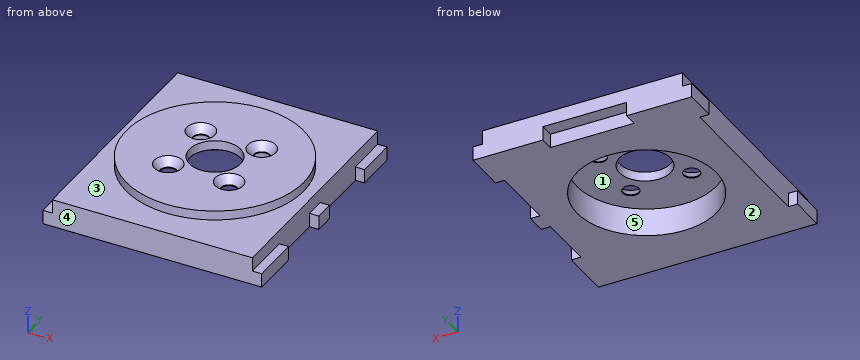
from build123d import *

# Parameters (mm, degrees)
F0_R     = 15
F1_DEPTH = 3
F2_R     = 15
F2_W     = 18
F2_H     = 3
F3_DEPTH = 3
F4_R     = 19.092503
F4_R_2   = 1.75
F4_R_3   = 5.5
F5_DEPTH = 2
F6_SIZE2 = 1.8
F6_SIZE  = 1.25
F7_W     = 2
F7_H     = 0.1
F8_DEPTH = 3.001


with BuildPart() as f1:
    # F0 (on Top) → F1 (new body)
    with BuildSketch(Plane.XY):
        Polygon((-9.5, 25.15), (-23.5, 25.15), (-23.5, 18.15), (-21.5, 18.15), (-21.5, -17.35), (-23.5, -17.35), (-23.5, -25.15), (23.5, -25.15), (23.5, -14.35), (21.5, -14.35), (21.5, -2.35), (23.5, -2.35), (23.5, 2.15), (21.5, 2.15), (21.5, 16.15), (23.5, 16.15), (23.5, 25.15), (8.5, 25.15), (8.5, 22.15), (-9.5, 22.15), align=None)
        with Locations((-0.135, -0.392646)):
            Circle(F0_R, mode=Mode.SUBTRACT)
    extrude(amount=F1_DEPTH)

    # F2 (on face) → F3 (join)
    with BuildSketch(Plane.XY.offset(3)):
        Polygon((-21.5, 25.15), (-21.5, 18.15), (-21.5, -17.35), (-21.5, -25.15), (21.5, -25.15), (21.5, -14.35), (21.5, -2.35), (21.5, 2.15), (21.5, 16.15), (21.5, 25.15), (8.5, 25.15), (8.5, 22.15), (-9.5, 22.15), (-9.5, 25.15), align=None)
        with Locations((-0.135, -0.392646)):
            Circle(F2_R, mode=Mode.SUBTRACT)
        with Locations((-0.5, 23.65)):
            Rectangle(F2_W, F2_H)
    extrude(amount=F3_DEPTH)

    # F4 (on face) → F5 (join)
    with BuildSketch(Plane.XY.offset(6)):
        Circle(F4_R)
        with Locations((-6.540738, -6.540738)):
            Circle(F4_R_2, mode=Mode.SUBTRACT)
        with Locations((6.540738, -6.540738)):
            Circle(F4_R_2, mode=Mode.SUBTRACT)
        with Locations((-6.540738, 6.540738)):
            Circle(F4_R_2, mode=Mode.SUBTRACT)
        Circle(F4_R_3, mode=Mode.SUBTRACT)
        with Locations((6.540738, 6.540738)):
            Circle(F4_R_2, mode=Mode.SUBTRACT)
    extrude(amount=F5_DEPTH)

    # F6
    f6_edges = [f1.edges().sort_by_distance(p)[0] for p in [
        (-8.290738, 6.540738, 8),
        (4.790738, 6.540738, 8),
        (4.790738, -6.540738, 8),
        (-8.290738, -6.540738, 8),
    ]]
    chamfer(f6_edges, length=F6_SIZE, length2=F6_SIZE2)

    # F7 (on face) → F8 (cut, through all)
    with BuildSketch(Plane.XY.offset(3)):
        with Locations((22.5, 2.1)):
            Rectangle(F7_W, F7_H)
        with Locations((22.5, -2.3)):
            Rectangle(F7_W, F7_H)
    extrude(amount=-F8_DEPTH, mode=Mode.SUBTRACT)


solid = f1.part
Read the model definition and answer for the solid it produces. Units are mm, in the model's axes. Face numbers are marked on the shaded views. A direction names the side the tool comes from. Coordinates: 2 decimals unless noted, no trailing zeros. Loops run counter-clockwise (first coordinate to the right, second up) from the corner with the lowest first, then second, coordinate; pieces in that order, holes last. Notation, with made-up numbers: (28.5, -12) - (49.5, -12) arc R30 cw to (49.5, 21) - close; hole circle Ø9 at (64.25, -25.5). An arc over 180 degrees is marked (long way). Answer in a Markdown table with one row per item.
Q1. Find section D-D on x = 0. Write down the section's boundary in (y, z).
Here are the results:
| item | result |
|---|---|
| outline | (-25.15, 0) - (-15.39, 0) - (-15.39, 6) - (-5.5, 6) - (-5.5, 8) - (-19.09, 8) - (-19.09, 6) - (-25.15, 6) - close; (5.5, 6) - (14.61, 6) - (14.61, 0) - (22.15, 0) - (22.15, 3) - (25.15, 3) - (25.15, 6) - (19.09, 6) - (19.09, 8) - (5.5, 8) - close |
Q2. Find section B-B on x = 11. Write down the section's boundary in (y, z).
Here are the results:
| item | result |
|---|---|
| outline | (-25.15, 0) - (-10.44, 0) - (-10.44, 6) - (9.66, 6) - (9.66, 0) - (25.15, 0) - (25.15, 6) - (15.61, 6) - (15.61, 8) - (-15.61, 8) - (-15.61, 6) - (-25.15, 6) - close |
Q3. Find section A-A on z = 0.75. Write down the section's boundary in (x, y) (3 decimals), plus the area to 3 significant figures.
Here are the results:
| item | result |
|---|---|
| outline | (-23.5, -25.15) - (23.5, -25.15) - (23.5, -14.35) - (21.5, -14.35) - (21.5, -2.25) - (23.5, -2.25) - (23.5, 2.05) - (21.5, 2.05) - (21.5, 16.15) - (23.5, 16.15) - (23.5, 25.15) - (8.5, 25.15) - (8.5, 22.15) - (-9.5, 22.15) - (-9.5, 25.15) - (-23.5, 25.15) - (-23.5, 18.15) - (-21.5, 18.15) - (-21.5, -17.35) - (-23.5, -17.35) - close; hole circle Ø30 at (-0.135, -0.393) |
| area | 1,480 mm^2 |
Q4. Given P1, Ø0.6, axis at x = 23, y = 0, coming from the +Z side; P2, Ø1, axis at x = -17.5, y = 16, coming from the -Z side; P3, Ø4.5, axis at x = 6.54, y = -6.54, coming from the +Z side; P4, Ø4, axis at y = 10.5, z = 3.5, coming from the -X side, each flat-ended and moving along its own axis, determine where each tip first touches the part or whether it passes through.
Here are the results:
| item | result |
|---|---|
| P1 | stops at z = 3 |
| P2 | stops at z = 0 |
| P3 | stops at z = 6.92 |
| P4 | stops at x = -21.5 |
Q5. Straight lines are drawn through the part: line 1 along Y through (x, z) = (8, 6.5); line 2 along X through (y, z) = (16, 1); line 3 along Z through (x, y) = (13, 0). For each, find the intervals that lie inside material, in ascending order. Write a range as [from, to].
Here are the results:
| item | result |
|---|---|
| line 1 | y = [-17.34, -7.85], [-5.23, 5.23], [7.85, 17.34] |
| line 2 | x = [-21.5, 21.5] |
| line 3 | z = [6, 8] |
Q6. The mould has two halves that part along X. Classify the marked faces 1 and 2: pulls with the +X half, pulls with the -X half, needs draft (parallel to the pull), parting line crosses it, or undercut.
Here are the results:
| item | result |
|---|---|
| face 1 | undercut |
| face 2 | needs draft |
Q7. Find section C-C on y = 13. Write down the section's boundary in (x, z).
Here are the results:
| item | result |
|---|---|
| outline | (-21.5, 0) - (-6.89, 0) - (-6.89, 6) - (6.62, 6) - (6.62, 0) - (21.5, 0) - (21.5, 6) - (13.98, 6) - (13.98, 8) - (-13.98, 8) - (-13.98, 6) - (-21.5, 6) - close |
Q8. For the marked faces 3, 4 and 5, determine the directions among +Z, -Z, +X, -X, +Y, -Y from which every point of the face is accessible in a straight line to the end or side of a thin tool.
Here are the results:
| item | result |
|---|---|
| face 3 | +Z |
| face 4 | +Z, -Z, +X, -X, -Y |
| face 5 | -Z |
